The model under review builds one solid part; all positions refer to its coordinate system, in mm. Face numbers are marked on the shaded views. A direction names the side the tool comes from. Round coordinates to 2 decimals unless told otherwise and drop trailing zeros. Order: outer loops, then holes, each group sorted by start corner. A loop starts at its lowest first (then second) coordinate and runs counter-clockwise, first axis right, second up. Notation, with made-up numbers: (23.25, -21.5) - (80.25, -21.5) arc R27 ccw to (80.25, -2.5) - close; hole circle Ø1 at (84, -26.75). An arc over 180 degrees is marked (long way). One line per question, with ' | ' between items. Start each with the question number.
Item 1: For L1, parallel to Z at x = 0, y = 1.5; L2, parallel to X at y = 2.05, z = 0; L3, parallel to X at y = 2.5, z = 7.5, list the stretches that pass through material, from the lowest coordinate up. Write a range as [from, to].
Item 2: Draft analysis for pull direction Z (two halves, no side actions). For the marked faces 4 and 5, state which applies: +Z half, -Z half, draft (parallel to the pull), parting line (faces both ways), or undercut.
Item 3: Add section C-C on x = 0. State how many separate pieces and enclosed holes the cut face has, and give its area (3 significant figures).
Item 4: Add section A-A on x = -55. State the section outline as (y, z) points.
Item 5: Tool access review of the marked faces 1, 2 and 3: name each direction out of +Z, -Z, +X, -X, +Y, -Y from which nothing blocks a thin tool from reaching the whole face with its end or side.
Item 6: Insertion check: pin 1 Ø1.9 at (x, z) = (55, 0) entering from +Y; pin 2 Ø2 at (y, z) = (19.5, -11) entering from +X; pin 3 Ø8 at (x, y) = (-36.5, 12) entering from -Z; pin 4 Ø5 at (x, z) = (0, -55) entering from +Y. Each pin has a flat end and moves straight along its axis. Give the tip position at first contact, or say it passes through.
Item 7: Add section B-B on z = -55. State the section outline as (x, y) points, and give its area (3 significant figures).
from build123d import *

# Parameters (mm, degrees)
SKETCH1_R           = 1.6
BOSS_EXTRUDE1_DEPTH = 3
CUT_EXTRUDE1_DEPTH  = 85.905830189
BOSS_EXTRUDE2_DEPTH = 2
BOSS_EXTRUDE3_DEPTH = 3
SHELL1_DEPTH        = 15
SHELL1_DRAFT        = 30.4655449
SKETCH6_W           = 10
SKETCH6_H           = 10
CUT_EXTRUDE2_DEPTH  = 88.177978871
CUT_EXTRUDE3_DEPTH  = 88.177978894
SKETCH8_W           = 151.222151061
SKETCH8_H           = 131.165318394
CUT_EXTRUDE4_DEPTH  = 1


# Read off the part's stored shape, not the designer's step: Shell1
with BuildPart() as part:
    # Sketch1 → Boss-Extrude1 (new body)
    with BuildSketch(Plane(origin=(0, 0, 0), x_dir=(1, 0, 0), z_dir=(0, 1, 0))):
        Polygon((24.852813742, 60), (-24.852813742, 60), (-60, 24.852813742), (-60, -24.852813742), (-24.852813742, -60), (24.852813742, -60), (60, -24.852813742), (60, 24.852813742), align=None)
        with Locations(Location((-38.890872965, -38.890872965, 0), (0, 0, 270))):
            Circle(SKETCH1_R, mode=Mode.SUBTRACT)
        with Locations(Location((0, -55, 0), (0, 0, 270))):
            Circle(SKETCH1_R, mode=Mode.SUBTRACT)
        with Locations(Location((38.890872965, -38.890872965, 0), (0, 0, 270))):
            Circle(SKETCH1_R, mode=Mode.SUBTRACT)
        with Locations(Location((38.890872965, 38.890872965, 0), (0, 0, 270))):
            Circle(SKETCH1_R, mode=Mode.SUBTRACT)
        with Locations(Location((0, 55, 0), (0, 0, 270))):
            Circle(SKETCH1_R, mode=Mode.SUBTRACT)
        with Locations(Location((-38.890872965, 38.890872965, 0), (0, 0, 270))):
            Circle(SKETCH1_R, mode=Mode.SUBTRACT)
        with Locations(Location((55, 0, 0), (0, 0, 270))):
            Circle(SKETCH1_R, mode=Mode.SUBTRACT)
        with Locations(Location((-55, 0, 0), (0, 0, 270))):
            Circle(SKETCH1_R, mode=Mode.SUBTRACT)
    extrude(amount=BOSS_EXTRUDE1_DEPTH)

    # Sketch2 → Cut-Extrude1 (cut, through all)
    with BuildSketch(Plane(origin=(0, 3, 0), x_dir=(1, 0, 0), z_dir=(0, 1, 0))):
        Polygon((20.710678119, 50), (-20.710678119, 50), (-50, 20.710678119), (-50, -20.710678119), (-20.710678119, -50), (20.710678119, -50), (50, -20.710678119), (50, 20.710678119), align=None)
    extrude(amount=-CUT_EXTRUDE1_DEPTH, mode=Mode.SUBTRACT)



with BuildPart() as body_2:
    # Sketch3 → Boss-Extrude2 (new body)
    with BuildSketch(Plane(origin=(0, 18, 0), x_dir=(1, 0, 0), z_dir=(0, 1, 0))):
        Polygon((16.568542495, 40), (-16.568542495, 40), (-40, 16.568542495), (-40, -16.568542495), (-16.568542495, -40), (16.568542495, -40), (40, -16.568542495), (40, 16.568542495), align=None)
    extrude(amount=BOSS_EXTRUDE2_DEPTH)

    # Sketch2<2> → section 0 of loft1
    with BuildSketch(Plane(origin=(0, 3, 0), x_dir=(1, 0, 0), z_dir=(0, 1, 0)), mode=Mode.PRIVATE) as loft1_s0:
        with BuildLine():
            Line((20.710678119, 50), (-20.710678119, 50))
            Line((-20.710678119, 50), (-50, 20.710678119))
            Line((-50, 20.710678119), (-50, -20.710678119))
            Line((-50, -20.710678119), (-20.710678119, -50))
            Line((-20.710678119, -50), (20.710678119, -50))
            Line((20.710678119, -50), (50, -20.710678119))
            Line((50, -20.710678119), (50, 20.710678119))
            Line((50, 20.710678119), (20.710678119, 50))
        make_face()
    # loft up to a face of the part (loft1)
    loft([loft1_s0.sketch, body_2.faces().sort_by_distance((0, 20, 0))[0]])


with BuildPart() as part_1:
    add(part.part)

    add(body_2.part)  # Boss-Extrude3 merges body 2
    # Sketch5 → Boss-Extrude3 (add)
    with BuildSketch(Plane.XZ.offset(-3)):
        Polygon((-50, -20.710678119), (-20.710678119, -50), (20.710678119, -50), (50, -20.710678119), (50, 20.710678119), (20.710678119, 50), (-20.710678119, 50), (-50, 20.710678119), align=None)
        Polygon((48, -19.882250994), (19.882250994, -48), (-19.882250994, -48), (-48, -19.882250994), (-48, 19.882250994), (-19.882250994, 48), (19.882250994, 48), (48, 19.882250994), align=None, mode=Mode.SUBTRACT)
    extrude(amount=BOSS_EXTRUDE3_DEPTH)


with BuildPart() as shell1_tool:
    # Shell1 outline → Shell1 (with draft: the straight prism first)
    with BuildSketch(Plane(origin=(0, 18, 0), x_dir=(1, 0, 0), z_dir=(0, 1, 0))):
        Polygon((16.09472687, 38.856107891), (-16.09472687, 38.856107891), (-38.856107891, 16.09472687), (-38.856107891, -16.09472687), (-16.09472687, -38.856107891), (16.09472687, -38.856107891), (38.856107891, -16.09472687), (38.856107891, 16.09472687), align=None)
    extrude(amount=-SHELL1_DEPTH)
    # Shell1: the draft: its side faces are tilted about the plane it starts from
    shell1_sides = [shell1_tool.faces().sort_by_distance(p)[0] for p in [
        (0, 10.5, -38.856107891),
        (-27.475417381, 10.5, -27.47541738),
        (-38.856107891, 10.5, 0),
        (-27.47541738, 10.5, 27.475417381),
        (0, 10.5, 38.856107891),
        (27.475417381, 10.5, 27.47541738),
        (38.856107891, 10.5, 0),
        (27.47541738, 10.5, -27.475417381),
    ]]
    draft(shell1_sides, Plane(origin=(0, 18, 0), x_dir=(1, 0, 0), z_dir=(0, 1, 0)), SHELL1_DRAFT)


with BuildPart() as part_2:
    add(part_1.part)

    # Shell1: cut by shell1_tool
    add(shell1_tool.part, mode=Mode.SUBTRACT)

    # Sketch6 → Cut-Extrude2 (cut, through all)
    with BuildSketch(Plane(origin=(0, 20, 0), x_dir=(1, 0, 0), z_dir=(0, 1, 0))):
        with Locations((0, 45)):
            Rectangle(SKETCH6_W, SKETCH6_H)
    extrude(amount=-CUT_EXTRUDE2_DEPTH, mode=Mode.SUBTRACT)

    # Sketch7 → Cut-Extrude3 (cut, through all)
    with BuildSketch(Plane(origin=(0, 20, 0), x_dir=(1, 0, 0), z_dir=(0, 1, 0))):
        with BuildLine():
            Line((-22, 26.533930893), (-22, -23.466069107))
            ThreePointArc((-22, -23.466069107), (-20, -25.466069107), (-18, -23.466069107))
            Line((-18, -23.466069107), (-18, 26.533930893))
            ThreePointArc((-18, 26.533930893), (-20, 28.533930893), (-22, 26.533930893))
        make_face()
        with BuildLine():
            Line((-28, 16.533930893), (-28, -13.466069107))
            ThreePointArc((-28, -13.466069107), (-30, -15.466069107), (-32, -13.466069107))
            Line((-32, -13.466069107), (-32, 16.533930893))
            ThreePointArc((-32, 16.533930893), (-30, 18.533930893), (-28, 16.533930893))
        make_face()
        with BuildLine():
            Line((-8, 31.533930893), (-8, -28.466069107))
            ThreePointArc((-8, -28.466069107), (-10, -30.466069107), (-12, -28.466069107))
            Line((-12, -28.466069107), (-12, 31.533930893))
            ThreePointArc((-12, 31.533930893), (-10, 33.533930893), (-8, 31.533930893))
        make_face()
        with BuildLine():
            Line((2, 31.533930893), (2, -28.466069107))
            ThreePointArc((2, -28.466069107), (0, -30.466069107), (-2, -28.466069107))
            Line((-2, -28.466069107), (-2, 31.533930893))
            ThreePointArc((-2, 31.533930893), (0, 33.533930893), (2, 31.533930893))
        make_face()
    cut_extrude3 = extrude(amount=-CUT_EXTRUDE3_DEPTH, mode=Mode.SUBTRACT)

    # Mirror1: Cut-Extrude3 across plane
    add(cut_extrude3.mirror(Plane.ZY), mode=Mode.SUBTRACT)

    # Sketch8 → Cut-Extrude4 (cut)
    with BuildSketch(Plane.XZ):
        with Locations((-0.059380878, -1.432630905)):
            Rectangle(SKETCH8_W, SKETCH8_H)
    extrude(amount=-CUT_EXTRUDE4_DEPTH, mode=Mode.SUBTRACT)


solid = part_2.part
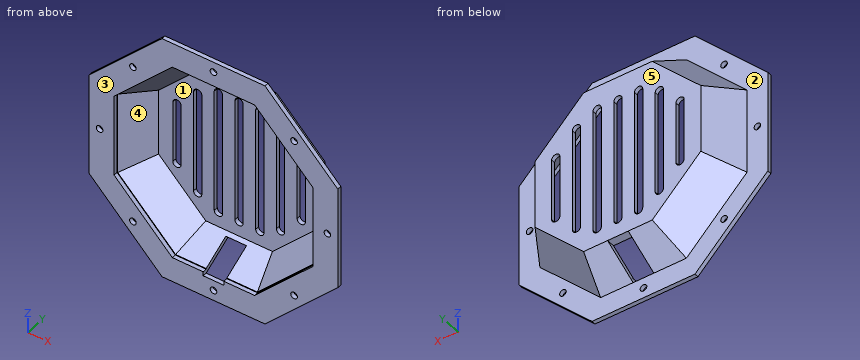
Determined:
1) L1: [-60, -56.6], [-53.4, -50], [48, 53.4], [56.6, 60] | L2: [-60, -56.6], [-53.4, -48], [48, 53.4], [56.6, 60] | L3: [-60, -48], [48, 60]
2) face 4: undercut | face 5: draft
3) separate pieces: 5 | enclosed holes: 0 | area: 100 mm2
4) outline: (1, -29.85) - (3, -29.85) - (3, -1.6) - (1, -1.6) - close; (1, 1.6) - (3, 1.6) - (3, 29.85) - (1, 29.85) - close
5) face 1: -Y | face 2: +Y | face 3: +Z, -Z, +X, -X, -Y
6) pin 1: through | pin 2: x = 40.88 | pin 3: z = -31.93 | pin 4: y = 3
7) outline: (-29.85, 1) - (-1.6, 1) - (-1.6, 3) - (-29.85, 3) - close; (1.6, 1) - (29.85, 1) - (29.85, 3) - (1.6, 3) - close | area: 113 mm2
